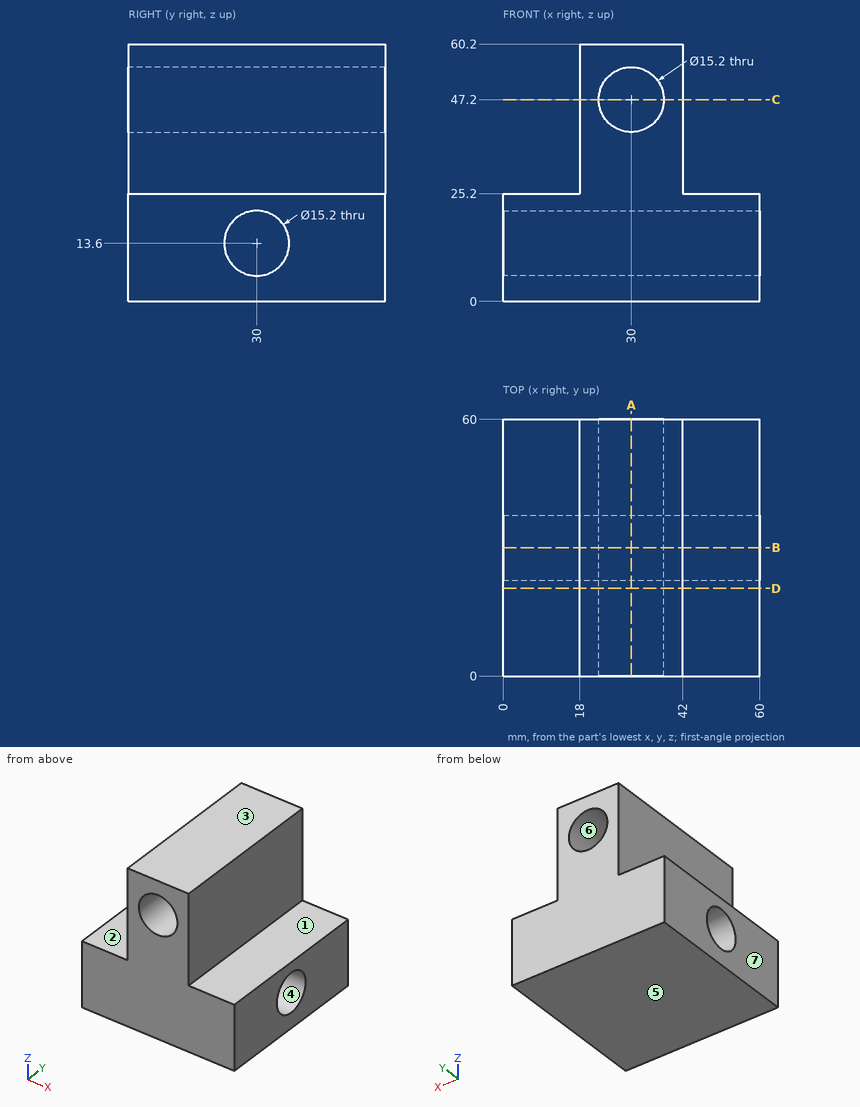
Study the drawing (mm; zero at the part's minimum x, y, z) and answer. A direction names the side the tool comes from. Give positions to 0.01 mm unless a question says otherwise; leave off trailing zeros. Write each loop counter-clockwise with the first axis right and the second up, starting at its lowest first coordinate (ties: lowest second). Pieces come first, ordered by that corner, then holes.
Item 1: Section C-C, the plane z = 47.2 is taken. Write down the section's boundary in (x, y).
Item 2: Find the intervals of material crossed by line 1 along X through (y, z) = (32.5, 47.2); line 2 along Y through (x, z) = (16, 13.6); line 3 along Z through (x, y) = (49, 11.5), in increasing order.
Item 3: Which of the six approach directions +Z, -Z, +X, -X, +Y, -Y give full straight-line access (tool end or side, diameter ignored) to the marked faces 1, 2 and 3?
Item 4: Section B-B, the plane y = 30 is taken. Write down the section's boundary in (x, z), plus the area to 3 significant figures.
Item 5: Determine the mould class of the marked faces 4, 5, 6 and 7 for opening direction Z: released by +Z, released by -Z, zero draft, split by the parting line, or undercut.
Item 6: Flat-ended cylindrical pins translate along their axes: P1, Ø4, axis at y = 34, z = 29, coming from the -X side; P2, Ø20, axis at x = 6.5, y = 22.5, coming from the +Z side; P3, Ø10.5, axis at y = 23.5, z = 36.5, coming from the +X side. Find the tip coordinate at first contact, or state that the pin passes through.
Item 7: Section A-A, the plane x = 30 is taken. Write down the section's boundary in (y, z).
Item 8: Section D-D, the plane y = 20.5 is taken. Write down the section's boundary in (x, z).
Completed:
1. outline: (18, 0) - (22.4, 0) - (22.4, 60) - (18, 60) - close; (37.6, 0) - (42, 0) - (42, 60) - (37.6, 60) - close
2. line 1: x = 18 to 22.4, 37.6 to 42
2. line 2: y = 0 to 22.4, 37.6 to 60
2. line 3: z = 0 to 25.2
3. face 1: +Z, +X, +Y, -Y
3. face 2: +Z, -X, +Y, -Y
3. face 3: +Z, +X, -X, +Y, -Y
4. outline: (0, 0) - (60, 0) - (60, 6) - (0, 6) - close; (0, 21.2) - (60, 21.2) - (60, 25.2) - (42, 25.2) - (42, 60.2) - (18, 60.2) - (18, 25.2) - (0, 25.2) - close; hole circle Ø15.2 at (30, 47.2)
4. area: 1,260 mm2
5. face 4: undercut
5. face 5: released by -Z
5. face 6: undercut
5. face 7: zero draft
6. P1: stops at x = 18
6. P2: stops at z = 25.2
6. P3: stops at x = 42
7. outline: (0, 0) - (60, 0) - (60, 39.6) - (0, 39.6) - close; (0, 54.8) - (60, 54.8) - (60, 60.2) - (0, 60.2) - close; hole circle Ø15.2 at (30, 13.6)
8. outline: (0, 0) - (60, 0) - (60, 25.2) - (42, 25.2) - (42, 60.2) - (18, 60.2) - (18, 25.2) - (0, 25.2) - close; hole circle Ø15.2 at (30, 47.2)
